For this review, take the finished solid that the model builds, in its own axes (mm). A direction names the side the tool comes from. Coordinates: 2 decimals unless noted, no trailing zeros. Write each loop counter-clockwise with the first axis right and the second up, starting at its lowest first coordinate (ties: lowest second). Pieces come first, ordered by that corner, then holes. Notation, with made-up numbers: (53.5, 62.5) - (86.5, 62.5) arc R22 cw to (86.5, 86.5) - close; hole circle Ø7 at (80.25, 43.25). An arc over 180 degrees is marked (long way). Use one line per item in the form item = value. Start each with the question number.
1) We need section D-D (y = -37). Give the boundary of the cut face in (x, z), plus the area to 3 significant figures.
2) Tool access review of faces 1 (the flat face through (-1, 49.032, 13)), 2 (the flat face through (-15, 14, 25.4)): name each direction out of +Z, -Z, +X, -X, +Y, -Y from which nothing blocks a thin tool from reaching the whole face with its end or side.
3) Insertion check: P1, Ø12, axis at x = 11.5, y = -7.5, coming from the +Z side; P2, Ø1.5, axis at y = -15, z = 32, coming from the +X side; P3, Ø3, axis at x = 14, y = -4, coming from the +Z side. Each pin has a flat end and moves straight along its axis. Give the tip position at first contact, or say it passes through.
4) We need section B-B (x = 0). Give the boundary of the cut face in (y, z), plus the area to 3 significant figures.
5) Mouldability with a two-part tool opening along X and no side actions: class faces 3 (the flat face through (-0.232, -0.232, 42.157)), 4 (the flat face through (-1, 3, 0)), 5 (the cylindrical face through (-16.534, 0.728, 35.1)), 6 (the flat face through (-60.305, 2, 13)) as pulls with the +X half, pulls with the -X half, needs draft (parallel to the pull), parting line crosses it, or undercut.
6) We need section A-A (y = 0). Give the boundary of the cut face in (x, z).
7) We need section C-C (z = 30). Give the boundary of the cut face in (x, y), plus the area to 3 significant figures.
8) For L1, parallel to Z at x = -52.5, y = 17.5; L2, parallel to X at y = -4, z = 29; L3, parallel to Y at x = -3.5, z = 37, list the stretches that pass through material, from the lowest coordinate up. Write a range as from..to.
```python
from build123d import *

# Parameters (mm, degrees)
F0_W     = 119.694226
F0_H     = 92.565984
F1_DEPTH = 25.4
F2_R     = 16.550029
F3_DEPTH = 25.4
F5_DEPTH = 92.566984


with BuildPart() as f1:
    # F0 (on Top) → F1 (new body)
    with BuildSketch(Plane.XY):
        with Locations((-0.458248, 2.749484)):
            Rectangle(F0_W, F0_H)
    extrude(amount=F1_DEPTH)

    # F2 (on face) → F3 (join)
    with BuildSketch(Plane.XY.offset(25.4)):
        Circle(F2_R)
    extrude(amount=F3_DEPTH)

    # F4 (on face) → F5 (cut, through all)
    with BuildSketch(Plane.XZ.offset(43.533508)):
        Polygon((16.550029, 50.8), (-16.550029, 50.8), (16.550029, 33.268765), align=None)
    extrude(amount=-F5_DEPTH, mode=Mode.SUBTRACT)


solid = f1.part
```
Determined:
q1.outline = (-60.31, 0) - (59.39, 0) - (59.39, 25.4) - (-60.31, 25.4) - close
q1.area = 3,040 mm²
q2.face_1 = +Z, -Z, +X, -X, +Y
q2.face_2 = +Z
q3.P1 = 39.12
q3.P2 = 8.42
q3.P3 = 35.41
q4.outline = (-43.53, 0) - (49.03, 0) - (49.03, 25.4) - (16.55, 25.4) - (16.55, 42.03) - (-16.55, 42.03) - (-16.55, 25.4) - (-43.53, 25.4) - close
q4.area = 2,900 mm²
q5.face_3 = pulls with the +X half
q5.face_4 = needs draft
q5.face_5 = parting line crosses it
q5.face_6 = pulls with the -X half
q6.outline = (-60.31, 0) - (59.39, 0) - (59.39, 25.4) - (16.55, 25.4) - (16.55, 33.27) - (-16.55, 50.8) - (-16.55, 25.4) - (-60.31, 25.4) - close
q7.outline = circle Ø33.1 at (0, 0)
q7.area = 860 mm²
q8.L1 = 0..25.4
q8.L2 = -16.06..16.06
q8.L3 = -16.18..16.18
